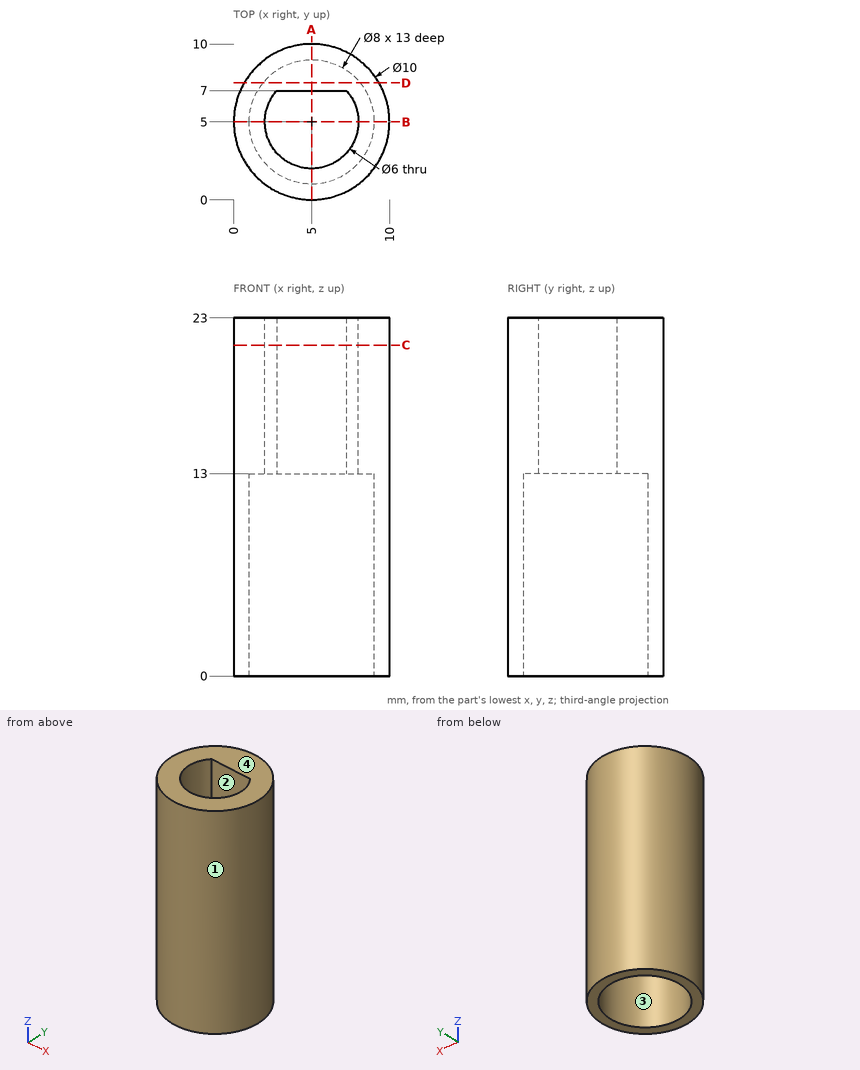
Study the drawing (mm; zero at the part's minimum x, y, z) and answer. Give positions to 0.01 mm unless a question says otherwise; leave off trailing zeros. Loops run counter-clockwise (first coordinate to the right, second up) from the corner with the lowest first, then second, coordinate; pieces in that order, holes last. Notation, with made-up numbers: (22, 37.25) -> (58, 37.25) arc R4 ccw to (58, 44.25) -> close; hole circle Ø11 at (-35.75, -31). An arc over 180 degrees is marked (long way). Write item = value, one per line. Start each with the question number.
(1) Find section B-B on y = 5. Give the vertices of the cut face in (x, z), and give its area (3 significant figures).
(2) Find section C-C on z = 21.25. Give the vertices of the cut face in (x, y).
(3) Given pin 1 Ø2.5 at (x, y) = (5, 6) entering from -Z; pin 2 Ø3 at (x, z) = (1.5, 11.5) entering from +Y; pin 3 Ø1.5 at (x, z) = (4, 10.5) entering from +Y, each flat-ended and moving along its own axis, determine where each tip first touches the part or whether it passes through.
(4) Find section A-A on x = 5. Give the vertices of the cut face in (y, z).
(5) The mould has two halves that part along Y. Classify the marked faces 1, 2, 3 and 4: +Y half, -Y half, draft (parallel to the pull), parting line (faces both ways), or undercut.
(6) Find section D-D on y = 7.5. Give the vertices of the cut face in (x, z).
(7) Find the intervals of material crossed by probe 1 along Y at (x, z) = (5, 5); probe 2 along Y at (x, z) = (5, 16); probe 3 along Z at (x, y) = (1.25, 4.75), in increasing order. Write a range as from..to.
From the geometry:
q1.outline = (0, 0) -> (1, 0) -> (1, 13) -> (2, 13) -> (2, 23) -> (0, 23) -> close; (8, 13) -> (9, 13) -> (9, 0) -> (10, 0) -> (10, 23) -> (8, 23) -> close
q1.area = 66.0 mm^2
q2.outline = circle Ø10 at (5, 5); hole (2.76, 7) arc R3 ccw (long way) to (7.24, 7) -> close
q3.pin_1 = 13
q3.pin_2 = 9.58
q3.pin_3 = 9.99
q4.outline = (0, 0) -> (1, 0) -> (1, 13) -> (2, 13) -> (2, 23) -> (0, 23) -> close; (7, 13) -> (9, 13) -> (9, 0) -> (10, 0) -> (10, 23) -> (7, 23) -> close
q5.face_1 = parting line
q5.face_2 = undercut
q5.face_3 = undercut
q5.face_4 = draft
q6.outline = (0.67, 0) -> (1.88, 0) -> (1.88, 13) -> (8.12, 13) -> (8.12, 0) -> (9.33, 0) -> (9.33, 23) -> (0.67, 23) -> close
q7.probe_1 = 0..1, 9..10
q7.probe_2 = 0..2, 7..10
q7.probe_3 = 13..23
